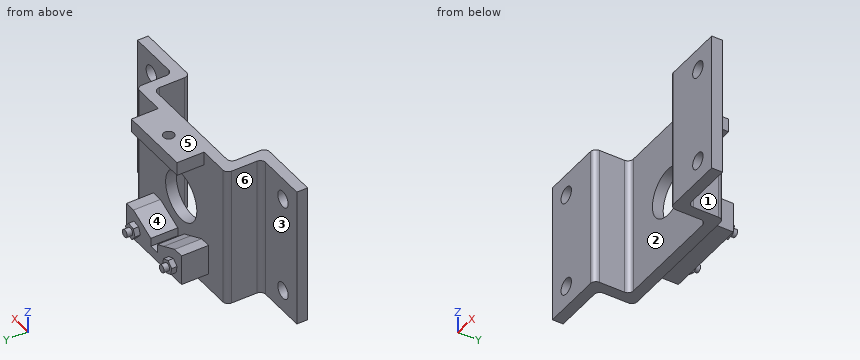
from build123d import *

# Parameters (mm, degrees)
EXTRUDE_1_DEPTH     = 130
FILLET_1_R          = 10
SKETCH_2_R          = 45
CUT_EXTRUDE_1_DEPTH = 260
SKETCH_3_R          = 7
EXTRUDE_2_DEPTH     = 50
SKETCH_4_R          = 7
EXTRUDE_3_DEPTH     = 10
SKETCH_5_R          = 7
EXTRUDE_4_DEPTH     = 70
SKETCH_6_W          = 132
SKETCH_6_H          = 25
EXTRUDE_5_DEPTH     = 50
SKETCH_7_R          = 10
CUT_EXTRUDE_2_DEPTH = 50
SKETCH_8_R          = 15
CUT_EXTRUDE_3_DEPTH = 30


with BuildPart() as part:
    # 草图1 → 凸台-拉伸1 (new body, symmetric)
    with BuildSketch(Plane.XY):
        Polygon((0, 0), (0, 20), (-130, 20), (-130, 10.839517471), (-130, -46.598965425), (-230, -46.598965425), (-230, -66.598965425), (-110, -66.598965425), (-110, 0), align=None)
        Polygon((130, 20), (0, 20), (0, 0), (110, 0), (110, -66.598965425), (230, -66.598965425), (230, -46.598965425), (130, -46.598965425), (130, 10.839517471), align=None)
    extrude(amount=EXTRUDE_1_DEPTH, both=True)

    # 圆角1
    fillet_1_edges = [part.edges().sort_by_distance(p)[0] for p in [
        (-130, 20, 0),
        (130, 20, 0),
        (130, -46.598965425, 0),
        (110, -66.598965425, 0),
        (110, 0, 0),
        (-110, 0, 0),
        (-110, -66.598965425, 0),
        (-130, -46.598965425, 0),
    ]]
    fillet(fillet_1_edges, radius=FILLET_1_R)

    # 草图2 → 切除-拉伸1 (cut)
    with BuildSketch(Plane(origin=(0, 20, 0), x_dir=(1, 0, 0), z_dir=(0, 1, 0))):
        Circle(SKETCH_2_R)
    extrude(amount=-CUT_EXTRUDE_1_DEPTH, mode=Mode.SUBTRACT)

    # 草图3 → 凸台-拉伸2 (add)
    with BuildSketch(Plane(origin=(0, 20, 0), x_dir=(1, 0, 0), z_dir=(0, 1, 0))):
        Polygon((79.997030901, 101.745041166), (0.475713007, 101.745041166), (0.475713007, 84.097255875), (9.839462373, 84.097255875), (9.839462373, 68.604224939), (59.997030901, 45.412205859), (79.997030901, 45.412205859), align=None)
        with Locations((53.744497978, 79.333035198)):
            Circle(SKETCH_3_R, mode=Mode.SUBTRACT)
        Polygon((-79.045604886, 45.412205859), (-59.045604886, 45.412205859), (-27.699569626, 59.906087225), (-8.888036358, 68.604224939), (-8.888036358, 84.097255875), (0.475713007, 84.097255875), (0.475713007, 101.745041166), (-79.045604886, 101.745041166), align=None)
        with Locations((-52.793071964, 79.333035198)):
            Circle(SKETCH_3_R, mode=Mode.SUBTRACT)
    extrude(amount=EXTRUDE_2_DEPTH)

    # 草图4 → 凸台-拉伸3 (add)
    with BuildSketch(Plane(origin=(0, 70, 0), x_dir=(1, 0, 0), z_dir=(0, 1, 0))):
        Polygon((48.795631933, 92.27555137), (40.061517162, 81.518449569), (45.010383207, 68.575933397), (58.693364024, 66.390519026), (67.427478795, 77.147620827), (62.47861275, 90.090136999), align=None)
        with Locations((53.744497978, 79.333035198)):
            Circle(SKETCH_4_R, mode=Mode.SUBTRACT)
        Polygon((-50.227927921, 92.949937784), (-63.303083503, 88.362966397), (-65.868227546, 74.746063811), (-55.358216006, 65.716132612), (-42.283060425, 70.303104), (-39.717916382, 83.920006586), align=None)
        with Locations((-52.793071964, 79.333035198)):
            Circle(SKETCH_4_R, mode=Mode.SUBTRACT)
    extrude(amount=EXTRUDE_3_DEPTH)

    # 草图5 → 凸台-拉伸4 (add)
    with BuildSketch(Plane(origin=(0, 20, 0), x_dir=(1, 0, 0), z_dir=(0, 1, 0))):
        with Locations((53.744497978, 79.333035198)):
            Circle(SKETCH_5_R)
        with Locations((-52.793071964, 79.333035198)):
            Circle(SKETCH_5_R)
    extrude(amount=EXTRUDE_4_DEPTH)

    # 草图6 → 凸台-拉伸5 (add)
    with BuildSketch(Plane(origin=(0, 20, 0), x_dir=(1, 0, 0), z_dir=(0, 1, 0))):
        with Locations((0, -117.5)):
            Rectangle(SKETCH_6_W, SKETCH_6_H)
    extrude(amount=EXTRUDE_5_DEPTH)

    # 草图7 → 切除-拉伸2 (cut)
    with BuildSketch(Plane.XY.offset(130)):
        with Locations((0, 43.080261377)):
            Circle(SKETCH_7_R)
    extrude(amount=-CUT_EXTRUDE_2_DEPTH, mode=Mode.SUBTRACT)

    # 草图8 → 切除-拉伸3 (cut)
    with BuildSketch(Plane(origin=(0, -46.598965425, 0), x_dir=(1, 0, 0), z_dir=(0, 1, 0))):
        with Locations((190, 90)):
            Circle(SKETCH_8_R)
        with Locations((190, -90)):
            Circle(SKETCH_8_R)
        with Locations((-190, -90)):
            Circle(SKETCH_8_R)
        with Locations((-190, 90)):
            Circle(SKETCH_8_R)
    extrude(amount=-CUT_EXTRUDE_3_DEPTH, mode=Mode.SUBTRACT)


solid = part.part
Verification items for the finished model (mm, model axes). Face numbers are marked on the shaded views. A direction names the side the tool comes from. Give positions to 0.01 mm unless a question says otherwise; leave off trailing zeros. Write each loop counter-clockwise with the first axis right and the second up, starting at its lowest first coordinate (ties: lowest second). Pieces come first, ordered by that corner, then holes. Notation, with made-up numbers: M -29.75,54.25 L -15.75,54.25 A27 ccw -15.75,73.25 Z; hole C 48,22.25 d2. An arc over 180 degrees is marked long. Put each result on its own line as item: value. Start each with the question number.
1. Section check A-A (x = -190). Record the cut outline in (y, z).
2. Draft check along Z on the marked faces 4, 5 and 6. Enter one of: +Z half, -Z half, draft (parallel to the pull), parting line (faces both ways), or undercut.
3. Scan lines: line 1 along Z through (x, y) = (190, -56); line 2 along X through (y, z) = (-54, 90); line 3 along X through (y, z) = (-50, -38.5). Record each from-to range of solid material in increasing order. Write a range as [from, to].
4. Section check B-B (z = 90). Record the cut outline in (x, y).
5. Section check D-D (z = 0). Record the cut outline in (x, y).
6. Go/stop test with flat-tipped pins: pin 1 Ø4 at (y, z) = (28, -55) entering from +X; pin 2 Ø22 at (x, y) = (74.5, 37.5) entering from +Z; pin 3 Ø15 at (y, z) = (53.5, -66.5) entering from -X; pin 4 Ø12.5 at (y, z) = (52, 122.5) entering from +X. Record where each tip stops, or that it passes through.
7. Section check C-C (y = -21). Record the cut outline in (x, z).
8. Set-up check for the marked faces 1, 2 and 3: record each of +Z, -Z, +X, -X, +Y, -Y from which the full face is reachable in a straight line by a thin tool's end or side.
Answer list:
1. outline: M -66.6,-130 L -46.6,-130 L -46.6,-105 L -66.6,-105 Z; M -66.6,-75 L -46.6,-75 L -46.6,75 L -66.6,75 Z; M -66.6,105 L -46.6,105 L -46.6,130 L -66.6,130 Z
2. face 4: undercut
2. face 5: +Z half
2. face 6: draft
3. line 1: [-130, -105], [-75, 75], [105, 130]
3. line 2: [-230, -205], [-175, -110], [110, 175], [205, 230]
3. line 3: [-230, -110], [110, 230]
4. outline: M -230,-66.6 L -205,-66.6 L -205,-46.6 L -230,-46.6 Z; M -175,-66.6 L -120,-66.6 A10 ccw -110,-56.6 L -110,-10 A10 cw -100,0 L 100,0 A10 cw 110,-10 L 110,-56.6 A10 ccw 120,-66.6 L 175,-66.6 L 175,-46.6 L 140,-46.6 A10 cw 130,-36.6 L 130,10 A10 ccw 120,20 L -120,20 A10 ccw -130,10 L -130,-36.6 A10 cw -140,-46.6 L -175,-46.6 Z; M 205,-66.6 L 230,-66.6 L 230,-46.6 L 205,-46.6 Z
5. outline: M -230,-66.6 L -120,-66.6 A10 ccw -110,-56.6 L -110,-10 A10 cw -100,0 L -45,0 L -45,20 L -120,20 A10 ccw -130,10 L -130,-36.6 A10 cw -140,-46.6 L -230,-46.6 Z; M 45,0 L 100,0 A10 cw 110,-10 L 110,-56.6 A10 ccw 120,-66.6 L 230,-66.6 L 230,-46.6 L 140,-46.6 A10 cw 130,-36.6 L 130,10 A10 ccw 120,20 L 45,20 Z
6. pin 1: x = 80
6. pin 2: z = 130
6. pin 3: x = -79.05
6. pin 4: x = 66
7. outline: M -130,-130 L -110,-130 L -110,130 L -130,130 Z; M 110,-130 L 130,-130 L 130,130 L 110,130 Z
8. face 1: +Z, -Z, +X, +Y
8. face 2: +Z, -Z, -Y
8. face 3: +Z, -Z, -X, +Y
